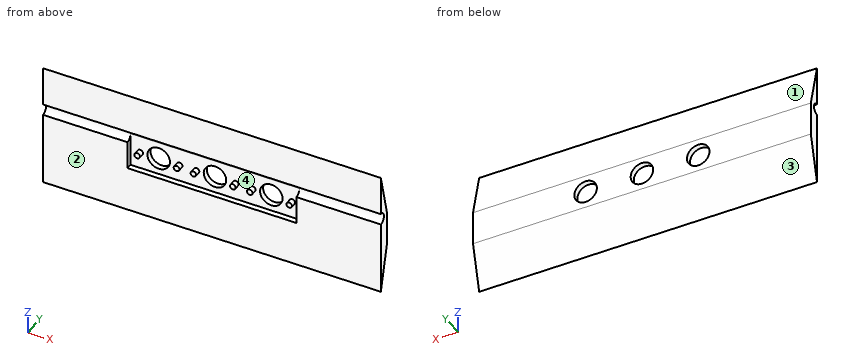
from build123d import *

# Parameters (mm, degrees)
BOSS_EXTRU_1_DEPTH      = 150
ESQUISSE3_R             = 5
ENL_V_MAT_EXTRU_1_DEPTH = 306.163890393
ESQUISSE5_R             = 10
ENL_V_MAT_EXTRU_2_DEPTH = 161.078105936
ESQUISSE6_W             = 150
ESQUISSE6_H             = 30
ESQUISSE6_R             = 2.5
ENL_V_MAT_EXTRU_3_DEPTH = 5


with BuildPart() as part:
    # Esquisse2 → Boss.-Extru.1 (new, symmetric)
    with BuildSketch(Plane(origin=(0, 0, 0), x_dir=(0, 0, -1), z_dir=(1, 0, 0))):
        Polygon((15, 0), (55, 0), (15, 10), (-15, 10), (-55, 0), (-15, 0), align=None)
    extrude(amount=BOSS_EXTRU_1_DEPTH, both=True)

    # Esquisse3 → Enlèv. mat.-Extru.1 (cut, through all)
    with BuildSketch(Plane.ZY.offset(150)):
        with Locations((15, 0)):
            Circle(ESQUISSE3_R)
    extrude(amount=-ENL_V_MAT_EXTRU_1_DEPTH, mode=Mode.SUBTRACT)

    # Esquisse5 → Enlèv. mat.-Extru.2 (cut, through all)
    with BuildSketch(Plane(origin=(0, 10, 0), x_dir=(1, 0, 0), z_dir=(0, 1, 0))):
        with Locations(Location((0, 0, 0), (0, 0, 270))):
            Circle(ESQUISSE5_R)
        with Locations(Location((50, 0, 0), (0, 0, 270))):
            Circle(ESQUISSE5_R)
        with Locations(Location((-50, 0, 0), (0, 0, 270))):
            Circle(ESQUISSE5_R)
    extrude(amount=-ENL_V_MAT_EXTRU_2_DEPTH, mode=Mode.SUBTRACT)

    # Esquisse6 → Enlèv. mat.-Extru.3 (cut)
    with BuildSketch(Plane.XZ):
        Rectangle(ESQUISSE6_W, ESQUISSE6_H)
        with Locations(Location((-66.424308402, 0, 0), (0, 0, 270))):
            Circle(ESQUISSE6_R, mode=Mode.SUBTRACT)
        with Locations(Location((-31.424308402, 0, 0), (0, 0, 270))):
            Circle(ESQUISSE6_R, mode=Mode.SUBTRACT)
        with Locations(Location((-16.424308402, 0, 0), (0, 0, 270))):
            Circle(ESQUISSE6_R, mode=Mode.SUBTRACT)
        with Locations(Location((18.575691598, 0, 0), (0, 0, 270))):
            Circle(ESQUISSE6_R, mode=Mode.SUBTRACT)
        with Locations(Location((33.575691598, 0, 0), (0, 0, 270))):
            Circle(ESQUISSE6_R, mode=Mode.SUBTRACT)
        with Locations(Location((68.575691598, 0, 0), (0, 0, 270))):
            Circle(ESQUISSE6_R, mode=Mode.SUBTRACT)
    extrude(amount=-ENL_V_MAT_EXTRU_3_DEPTH, mode=Mode.SUBTRACT)


solid = part.part
Read the model definition and answer for the solid it produces. Units are mm, in the model's axes. Face numbers are marked on the shaded views. Coordinates: 2 decimals unless noted, no trailing zeros. Order: outer loops, then holes, each group sorted by start corner. A loop starts at its lowest first (then second) coordinate and runs counter-clockwise, first axis right, second up. Notation, with made-up numbers: M -32.5,29.25 L -24.5,29.25 A27 ccw -24.5,46.25 Z; hole C 39,-3.75 d2. An arc over 180 degrees is marked long. Put each result on its own line as item: value. Start each with the question number.
Item 1: The mould has two halves that part along Z. Classify the marked faces 1, 2, 3 and 4: +Z half, -Z half, draft (parallel to the pull), parting line (faces both ways), or undercut.
Item 2: Section D-D, the plane x = 47 is taken. Determine the outline of the cut face in (y, z).
Item 3: Given pin 1 Ø23 at (x, z) = (50, 0) entering from +Y; pin 2 Ø12 at (x, z) = (82, -33.5) entering from +Y (3 decimals); pin 3 Ø3 at (x, z) = (28, 17) entering from +Y (3 decimals), each flat-ended and moving along its own axis, determine where each tip first touches the part or whether it passes through.
Item 4: Consider probe 1 along X at (y, z) = (6.35, 0); probe 2 along X at (y, z) = (2.5, -12); probe 3 along X at (y, z) = (9, -1.5). Determine where each line is inside the solid, lowest interval first. Write a range as [from, to].
Item 5: Section B-B, the plane y = 6.5 is taken. Determine the outline of the cut face in (x, z).
Item 6: Section C-C, the plane z = 36 is taken. Determine the outline of the cut face in (x, y), plus the area to 4 significant figures.
Item 7: Section A-A, the plane x = 0 is taken. Determine the outline of the cut face in (y, z), plus the area to 3 significant figures.
Computed:
1. face 1: +Z half
1. face 2: draft
1. face 3: -Z half
1. face 4: undercut
2. outline: M 0,-55 L 10,-15 L 10,-9.54 L 5,-9.54 L 5,-15 L 0,-15 Z; M 0,20 A5 cw 5,15 L 5,9.54 L 10,9.54 L 10,15 L 0,55 Z
3. pin 1: stops at y = 10
3. pin 2: stops at y = 6.875
3. pin 3: stops at y = 9.875
4. probe 1: x = [-150, -60], [-40, -10], [10, 40], [60, 150]
4. probe 2: x = [-150, -75], [75, 150]
4. probe 3: x = [-150, -59.89], [-40.11, -9.89], [9.89, 40.11], [59.89, 150]
5. outline: M -150,-29 L 150,-29 L 150,29 L -150,29 Z; hole C -50,0 d20; hole C 0,0 d20; hole C 50,0 d20
6. outline: M -150,0 L 150,0 L 150,4.75 L -150,4.75 Z
6. area: 1,425 mm2
7. outline: M 0,-55 L 10,-15 L 10,-10 L 5,-10 L 5,-15 L 0,-15 Z; M 0,20 A5 cw 5,15 L 5,10 L 10,10 L 10,15 L 0,55 Z
7. area: 430 mm2
